from build123d import *

# Parameters (mm, degrees)
F0_W      = 210
F0_H      = 85
F1_DEPTH  = 5
F2_R      = 10
F4_DEPTH  = 4
F6_DEPTH  = 3
F8_DEPTH  = 3
F9_R      = 3
F10_DEPTH = 25
F11_R     = 8
F12_DEPTH = 4.1
F14_DEPTH = 25


with BuildPart() as f1:
    # F0 (on Top) → F1 (new body)
    with BuildSketch(Plane.XY):
        Rectangle(F0_W, F0_H)
    extrude(amount=F1_DEPTH)

    # F2
    f2_edges = [f1.edges().sort_by_distance(p)[0] for p in [
        (-105, -42.5, 2.5),
        (-105, 42.5, 2.5),
        (105, 42.5, 2.5),
        (105, -42.5, 2.5),
    ]]
    fillet(f2_edges, radius=F2_R)

    # F3 (on face) → F4 (join)
    with BuildSketch(Plane.XY.offset(5)):
        with BuildLine():
            Line((66, 41), (-66, 41))
            ThreePointArc((-66, 41), (-69.535534, 39.535534), (-71, 36))
            Line((-71, 36), (-71, -36))
            ThreePointArc((-71, -36), (-69.535534, -39.535534), (-66, -41))
            Line((-66, -41), (66, -41))
            ThreePointArc((66, -41), (69.535534, -39.535534), (71, -36))
            Line((71, -36), (71, 36))
            ThreePointArc((71, 36), (69.535534, 39.535534), (66, 41))
        make_face()
    extrude(amount=F4_DEPTH)

    # F5 (on face) → F6 (cut)
    with BuildSketch(Plane.XY.offset(9)):
        with BuildLine():
            Line((62, 39), (-62, 39))
            ThreePointArc((-62, 39), (-65.535534, 37.535534), (-67, 34))
            Line((-67, 34), (-67, -34))
            ThreePointArc((-67, -34), (-65.535534, -37.535534), (-62, -39))
            Line((-62, -39), (62, -39))
            ThreePointArc((62, -39), (65.535534, -37.535534), (67, -34))
            Line((67, -34), (67, 34))
            ThreePointArc((67, 34), (65.535534, 37.535534), (62, 39))
        make_face()
    extrude(amount=-F6_DEPTH, mode=Mode.SUBTRACT)

    # F7 (on face) → F8 (join)
    with BuildSketch(Plane.XY.offset(6)):
        with BuildLine():
            Line((52, 34), (-52, 34))
            Line((-52, 34), (-52, 27))
            ThreePointArc((-52, 27), (-52.87868, 24.87868), (-55, 24))
            Line((-55, 24), (-62, 24))
            Line((-62, 24), (-62, -24))
            Line((-62, -24), (-55, -24))
            ThreePointArc((-55, -24), (-52.87868, -24.87868), (-52, -27))
            Line((-52, -27), (-52, -34))
            Line((-52, -34), (52, -34))
            Line((52, -34), (52, -27))
            ThreePointArc((52, -27), (52.87868, -24.87868), (55, -24))
            Line((55, -24), (62, -24))
            Line((62, -24), (62, 24))
            Line((62, 24), (55, 24))
            ThreePointArc((55, 24), (52.87868, 24.87868), (52, 27))
            Line((52, 27), (52, 34))
        make_face()
    extrude(amount=F8_DEPTH)

    # F9 (on face) → F10 (cut)
    with BuildSketch(Plane.XY.offset(6)):
        with Locations((-61, -33)):
            Circle(F9_R)
        with Locations((-61, 33)):
            Circle(F9_R)
        with Locations((61, -33)):
            Circle(F9_R)
        with Locations((61, 33)):
            Circle(F9_R)
    extrude(amount=-F10_DEPTH, mode=Mode.SUBTRACT)

    # F11 (on face) → F12 (cut)
    with BuildSketch(Plane(origin=(0, 0, 0), x_dir=(1, 0, 0), z_dir=(0, 0, -1))):
        with Locations((-61, 33)):
            Circle(F11_R)
        with Locations((-61, -33)):
            Circle(F11_R)
        with Locations((61, -33)):
            Circle(F11_R)
        with Locations((61, 33)):
            Circle(F11_R)
    extrude(amount=-F12_DEPTH, mode=Mode.SUBTRACT)

    # F13 (on face) → F14 (cut)
    with BuildSketch(Plane.XY.offset(5)):
        with BuildLine():
            Line((-80, 32.5), (-90, 32.5))
            ThreePointArc((-90, 32.5), (-93.535534, 31.035534), (-95, 27.5))
            Line((-95, 27.5), (-95, 7.5))
            Line((-95, 7.5), (-75, 7.5))
            Line((-75, 7.5), (-75, 27.5))
            ThreePointArc((-75, 27.5), (-76.464466, 31.035534), (-80, 32.5))
        make_face()
        with BuildLine():
            ThreePointArc((-80, -32.5), (-76.464466, -31.035534), (-75, -27.5))
            Line((-75, -27.5), (-75, -7.5))
            Line((-75, -7.5), (-95, -7.5))
            Line((-95, -7.5), (-95, -27.5))
            ThreePointArc((-95, -27.5), (-93.535534, -31.035534), (-90, -32.5))
            Line((-90, -32.5), (-80, -32.5))
        make_face()
        with BuildLine():
            ThreePointArc((80, 32.5), (76.464466, 31.035534), (75, 27.5))
            Line((75, 27.5), (75, 7.5))
            Line((75, 7.5), (95, 7.5))
            Line((95, 7.5), (95, 27.5))
            ThreePointArc((95, 27.5), (93.535534, 31.035534), (90, 32.5))
            Line((90, 32.5), (80, 32.5))
        make_face()
        with BuildLine():
            Line((75, -7.5), (75, -27.5))
            ThreePointArc((75, -27.5), (76.464466, -31.035534), (80, -32.5))
            Line((80, -32.5), (90, -32.5))
            ThreePointArc((90, -32.5), (93.535534, -31.035534), (95, -27.5))
            Line((95, -27.5), (95, -7.5))
            Line((95, -7.5), (75, -7.5))
        make_face()
    extrude(amount=-F14_DEPTH, mode=Mode.SUBTRACT)


solid = f1.part
Design review of the part built by this model. Coordinates are the model's own, in mm. A direction names the side the tool comes from. Coordinates: 2 decimals unless noted, no trailing zeros. Loops run counter-clockwise (first coordinate to the right, second up) from the corner with the lowest first, then second, coordinate; pieces in that order, holes last. Notation, with made-up numbers: (-20.5, 3) -> (36.5, 3) arc R19 ccw to (36.5, 40) -> close; hole circle Ø5 at (35, 82). An arc over 180 degrees is marked (long way). Use a Markdown table: item, result. Add a question column.
Item 1: Machinability: for faces 1 (the cylindrical face through (55.1, 27.6, 2)), 2 (the cylindrical face through (66, 37, 8)), 3 (the cylindrical face through (-69, 40, 7)), 4 (the flat face through (-71, 1, 7)), 5 (the flat face through (-85, 7.5, 3)), which of the approach directions +Z, -Z, +X, -X, +Y, -Y give a long, thin tool a straight path to every point of the face, cutting with its end or side? Answer none if there is none.
Item 2: We need section B-B, the plane x = -34. Write out the cut boundary in (y, z), and give its area (3 significant figures).
Item 3: The part is to be moulded in two halves that separate along Y. For faces 6 (the cylindrical face through (-62.041, -40.932, 2.021)), 7 (the cylindrical face through (-102.15, 39.49, 2.54)), 8 (the cylindrical face through (69, -40, 7)), 9 (the flat face through (85, -7.5, 3)), say which applies: +Y half, -Y half, draft (parallel to the pull), parting line (faces both ways), or undercut.
Item 4: Wall thickness on L1, parallel to X at y = -15, z = 7.5; L2, parallel to X at y = -23.5, z = 0.5; L3, parallel to Y at x = -61, z = 4.8: over which ranges is each line inside the solid? List them lowest first. Write a range as from..to.
Item 5: Clearance check with flat-ended pins moving along their axes: P1, Ø4.5, axis at y = -11.5, z = 7, coming from the +X side; P2, Ø1.5, axis at y = -30, z = 7.5, coming from the +X side; P3, Ø5.5, axis at x = -61, y = 33, coming from the -Z side; P4, Ø9.5, axis at x = 61, y = 33, coming from the +Z side. State where each tip first meets the part, or that it passes through.
Item 6: We need section A-A, the plane y = 10. Write out the cut boundary in (x, z), and give its area (3 significant figures).
Numbers:
| question | item | result |
|---|---|---|
| 1 | face 1 | -Z |
| 1 | face 2 | +Z |
| 1 | face 3 | +Z, -X, +Y |
| 1 | face 4 | +Z, -X, +Y, -Y |
| 1 | face 5 | +Z, -Z |
| 2 | outline | (-42.5, 0) -> (42.5, 0) -> (42.5, 5) -> (41, 5) -> (41, 9) -> (39, 9) -> (39, 6) -> (34, 6) -> (34, 9) -> (-34, 9) -> (-34, 6) -> (-39, 6) -> (-39, 9) -> (-41, 9) -> (-41, 5) -> (-42.5, 5) -> close |
| 2 | area | 723 mm^2 |
| 3 | face 6 | undercut |
| 3 | face 7 | +Y half |
| 3 | face 8 | -Y half |
| 3 | face 9 | undercut |
| 4 | L1 | x = -71..-67, -62..62, 67..71 |
| 4 | L2 | x = -105..-95, -75..75, 95..105 |
| 4 | L3 | y = -42.5..-36, -30..30, 36..42.5 |
| 5 | P1 | stops at x = 105 |
| 5 | P2 | stops at x = 71 |
| 5 | P3 | passes through |
| 5 | P4 | stops at z = 6 |
| 6 | outline | (-105, 0) -> (-95, 0) -> (-95, 5) -> (-105, 5) -> close; (-75, 0) -> (75, 0) -> (75, 5) -> (71, 5) -> (71, 9) -> (67, 9) -> (67, 6) -> (62, 6) -> (62, 9) -> (-62, 9) -> (-62, 6) -> (-67, 6) -> (-67, 9) -> (-71, 9) -> (-71, 5) -> (-75, 5) -> close; (95, 0) -> (105, 0) -> (105, 5) -> (95, 5) -> close |
| 6 | area | 1,390 mm^2 |
